The model under review builds one solid part; all positions refer to its coordinate system, in mm. A direction names the side the tool comes from. Round coordinates to 2 decimals unless told otherwise and drop trailing zeros. Order: outer loops, then holes, each group sorted by start corner. A loop starts at its lowest first (then second) coordinate and runs counter-clockwise, first axis right, second up. Notation, with made-up numbers: M -37,72 L -17,72 A24 ccw -17,93 Z; hole C -21,65.5 d10. An arc over 180 degrees is marked long. Answer as CSV lines item,"result". Start each with the question number.
from build123d import *

# Parameters (mm, degrees)
SKETCH011_R     = 1.7
PAD007_DEPTH    = 2
SKETCH012_W     = 3
SKETCH012_H     = 12.5
PAD008_DEPTH    = 21
SKETCH013_R     = 1.4
POCKET004_DEPTH = 5
FILLET007_R     = 5
CHAMFER003_SIZE = 1.499
CHAMFER004_SIZE = 2.9999
CHAMFER005_SIZE = 0.5


with BuildPart() as part:
    # Sketch011 → Pad007 (new body)
    with BuildSketch(Plane.XY):
        with BuildLine():
            Line((0, -4), (4.7, -4))
            Line((4.7, -7), (4.7, -4))
            Line((7.7, -7), (4.7, -7))
            Line((7.7, -7), (7.7, 5.5))
            Line((4.7, 5.5), (7.7, 5.5))
            Line((4.7, 4), (4.7, 5.5))
            Line((4.7, 4), (0, 4))
            ThreePointArc((0, 4), (-4, 0), (0, -4))
        make_face()
        Circle(SKETCH011_R, mode=Mode.SUBTRACT)
    extrude(amount=PAD007_DEPTH)

    # Sketch012 (on Face11 of Pad007) → Pad008 (join)
    with BuildSketch(Plane.XY.offset(2)):
        with Locations((6.2, -0.75)):
            Rectangle(SKETCH012_W, SKETCH012_H)
    extrude(amount=PAD008_DEPTH)

    # Sketch013 (on Face7 of Pad008) → Pocket004 (cut)
    with BuildSketch(Plane(origin=(4.7, 0, 0), x_dir=(0, -1, 0), z_dir=(-1, 0, 0))):
        with Locations((1.05, 20)):
            Circle(SKETCH013_R)
    extrude(amount=-POCKET004_DEPTH, mode=Mode.SUBTRACT)

    # Fillet007
    fillet007_edges = [part.edges().sort_by_distance(p)[0] for p in [
        (6.2, 5.5, 23),
        (6.2, -7, 23),
    ]]
    fillet(fillet007_edges, radius=FILLET007_R)

    # Chamfer003
    chamfer003_edges = [part.edges().sort_by_distance(p)[0] for p in [
        (4.7, 4, 1),
    ]]
    chamfer(chamfer003_edges, length=CHAMFER003_SIZE)

    # Chamfer004
    chamfer004_edges = [part.edges().sort_by_distance(p)[0] for p in [
        (4.7, -4, 1),
    ]]
    chamfer(chamfer004_edges, length=CHAMFER004_SIZE)

    # Chamfer005
    chamfer005_edges = [part.edges().sort_by_distance(p)[0] for p in [
        (7.7, 5.5, 10),
    ]]
    chamfer(chamfer005_edges, length=CHAMFER005_SIZE)


with BuildPart() as part_1:
    # Body006 placement: moved
    add(part.part.moved(Location((33, -46, 3))))


solid = part_1.part
Item 1: Consider section A-A (y = -46). State the section outline as (x, z) points.
Item 2: Wall thickness on probe 1 along Y at (x, z) = (33, 3.4); probe 2 along Z at (x, y) = (39.35, -47.05); probe 3 along Z at (x, y) = (34.5, -47.75): over which ranges is each line inside the solid? List them lowest first. Write a range as [from, to].
Item 3: Consider section D-D (x = 34). State the section outline as (y, z) points.
Item 4: For pin 1 (6 mm diameter, centred on y = -47, z = 23, fed in from -X); pin 2 (4.5 mm diameter, centred on x = 33.5, y = -46.5, fed in from +Z); pin 3 (1.4 mm diameter, centred on x = 33.5, z = 3.5, fed in from -Y), all flat-tipped, find the tip position at first contact; note any pin that passes through.
Item 5: Consider section C-C (z = 5.5). State the section outline as (x, y) points.
Item 6: Tool access review of faces 4 (the flat face through (34, -50, 4)), 5 (the conical face through (40.558, -51.319, 24.246)), 6 (the cylindrical face through (39, -51, 25)), 7 (the flat face through (35, -42, 4)), 8 (the flat face through (37.7, -47, 14)): name each direction out of +Z, -Z, +X, -X, +Y, -Y from which nothing blocks a thin tool from reaching the whole face with its end or side.
Item 7: Consider section B-B (x = 38.25). State the section outline as (y, z) points.
Item 8: The part is to be moulded in two halves that separate along Y. For faces 1 (the cylindrical face through (39.18, -45.94, 22.15)), 2 (the flat face through (36.9, -41.3, 4)), 3 (the flat face through (36, -47, 3)), say which applies: +Y half, -Y half, draft (parallel to the pull), parting line (faces both ways), or undercut.
Reported:
1,outline,"M 29,3 L 31.3,3 L 31.3,5 L 29,5 Z; M 34.7,3 L 40.7,3 L 40.7,22.07 L 37.7,22.07 L 37.7,5 L 34.7,5 Z; M 37.7,23.93 L 40.7,23.93 L 40.7,25.5 L 40.2,26 L 37.7,26 Z"
2,probe 1,"y = [-50, -47.7], [-44.3, -42]"
2,probe 2,"z = [3, 21.6], [24.4, 26]"
2,probe 3,"z = [3, 5]"
3,outline,"M -50,3 L -47.37,3 L -47.37,5 L -50,5 Z; M -44.63,3 L -42,3 L -42,5 L -44.63,5 Z"
4,pin 1,"stops at x = 37.7"
4,pin 2,"stops at z = 5"
4,pin 3,"stops at y = -50"
5,outline,"M 37.7,-53 L 40.2,-53 L 40.7,-52.5 L 40.7,-41 L 40.2,-40.5 L 37.7,-40.5 Z"
6,face 4,"+Z, -Z, -X, -Y"
6,face 5,"+Z, +X, -Y"
6,face 6,"+Z, +X, -X, -Y"
6,face 7,"+Z, -Z, -X, +Y"
6,face 8,"+Z, -X, +Y, -Y"
7,outline,"M -53,3 L -40.5,3 L -40.5,21 A5 ccw -45.5,26 L -48,26 A5 ccw -53,21 Z; hole C -47.05,23 d2.8"
8,face 1,"undercut"
8,face 2,"+Y half"
8,face 3,"draft"
